from build123d import *

# Parameters (mm, degrees)
SKETCH1_W           = 75
SKETCH1_H           = 45
SKETCH1_R           = 14
SKETCH1_R_2         = 1.6
BOSS_EXTRUDE1_DEPTH = 2.032
FILLET2_R           = 5
SKETCH2_R           = 1.6
CUT_EXTRUDE1_DEPTH  = 3.032
SKETCH3_R           = 1.6
CUT_EXTRUDE2_DEPTH  = 3.032


with BuildPart() as part:
    # Sketch1 → Boss-Extrude1 (new body)
    with BuildSketch(Plane.XY):
        Rectangle(SKETCH1_W, SKETCH1_H)
        Circle(SKETCH1_R, mode=Mode.SUBTRACT)
        with Locations((-15.5, 15.5)):
            Circle(SKETCH1_R_2, mode=Mode.SUBTRACT)
        with Locations((15.5, 15.5)):
            Circle(SKETCH1_R_2, mode=Mode.SUBTRACT)
        with Locations((15.5, -15.5)):
            Circle(SKETCH1_R_2, mode=Mode.SUBTRACT)
        with Locations((-15.5, -15.5)):
            Circle(SKETCH1_R_2, mode=Mode.SUBTRACT)
    extrude(amount=BOSS_EXTRUDE1_DEPTH)

    # Fillet2
    fillet2_edges = [part.edges().sort_by_distance(p)[0] for p in [
        (37.5, -22.5, 1.016),
        (-37.5, -22.5, 1.016),
        (-37.5, 22.5, 1.016),
        (37.5, 22.5, 1.016),
    ]]
    fillet(fillet2_edges, radius=FILLET2_R)

    # Sketch2 → Cut-Extrude1 (cut, through all)
    with BuildSketch(Plane.XY.offset(2.032)):
        with Locations((-30, 0)):
            Circle(SKETCH2_R)
        with Locations((-30, 15)):
            Circle(SKETCH2_R)
        with Locations((-30, -15)):
            Circle(SKETCH2_R)
        with Locations((30, -15)):
            Circle(SKETCH2_R)
        with Locations((30, 15)):
            Circle(SKETCH2_R)
        with Locations((30, 0)):
            Circle(SKETCH2_R)
    extrude(amount=-CUT_EXTRUDE1_DEPTH, mode=Mode.SUBTRACT)

    # Sketch3 → Cut-Extrude2 (cut, through all)
    with BuildSketch(Plane(origin=(0, 0, 0), x_dir=(-1, 0, 0), z_dir=(0, 0, -1))):
        with Locations((-32.5, 5)):
            Circle(SKETCH3_R)
        with Locations((-32.5, -5)):
            Circle(SKETCH3_R)
        with Locations((32.5, -5)):
            Circle(SKETCH3_R)
        with Locations((32.5, 5)):
            Circle(SKETCH3_R)
    extrude(amount=-CUT_EXTRUDE2_DEPTH, mode=Mode.SUBTRACT)


solid = part.part
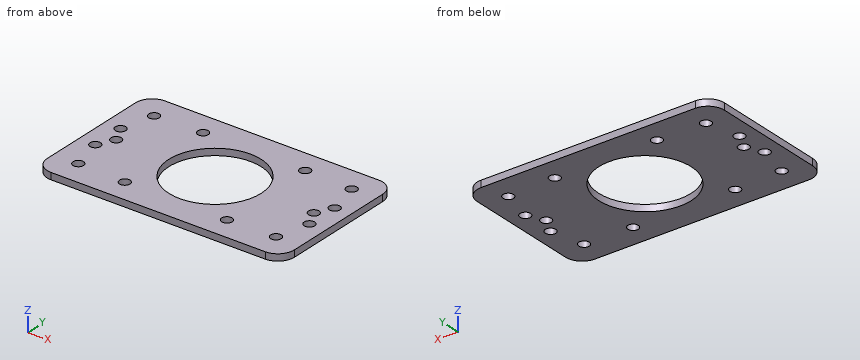
Geometry check sheet. Reference: the model listing, model coordinates, mm. Give positions to 0.01 mm unless a question says otherwise; leave off trailing zeros. Write each loop counter-clockwise with the first axis right and the second up, starting at its lowest first coordinate (ties: lowest second). Pieces come first, ordered by that corner, then holes. Notation, with made-up numbers: (-37.5, 23.25) - (-9.5, 23.25) arc R11 ccw to (-9.5, 34.25) - close; hole circle Ø8 at (72, 30.5). An arc over 180 degrees is marked (long way). Put each result on its own line as item: value.
1. Go/stop test with a flat-tipped pin: pin 1 (3 mm diameter, centred on x = 30, y = 0, fed in from +Z). Record where the tip stops, or that it passes through.
Ans:
pin 1: passes through
2. Sectioned sample at B-B, the plane x = 15.5. Enter the section's corners in (y, z).
Ans:
outline: (-22.5, 0) - (-17.1, 0) - (-17.1, 2.03) - (-22.5, 2.03) - close; (-13.9, 0) - (13.9, 0) - (13.9, 2.03) - (-13.9, 2.03) - close; (17.1, 0) - (22.5, 0) - (22.5, 2.03) - (17.1, 2.03) - close
3. Sectioned sample at A-A, the plane y = 0. Enter the section's corners in (x, z), plus the area to 3 significant figures.
Ans:
outline: (-37.5, 0) - (-31.6, 0) - (-31.6, 2.03) - (-37.5, 2.03) - close; (-28.4, 0) - (-14, 0) - (-14, 2.03) - (-28.4, 2.03) - close; (14, 0) - (28.4, 0) - (28.4, 2.03) - (14, 2.03) - close; (31.6, 0) - (37.5, 0) - (37.5, 2.03) - (31.6, 2.03) - close
area: 82.5 mm²
4. Thickness scan on line 1 (Y direction, x = -15.5, z = 0.7); line 2 (Y direction, x = -32.5, z = 1.1); line 3 (Y direction, x = 0, z = 0.6). Record the ranges inside material, lowest first.
Ans:
line 1: y = -22.5 to -17.1, -13.9 to 13.9, 17.1 to 22.5
line 2: y = -22.5 to -6.6, -3.4 to 3.4, 6.6 to 22.5
line 3: y = -22.5 to -14, 14 to 22.5
5. Sectioned sample at C-C, the plane x = 0. Enter the section's corners in (y, z).
Ans:
outline: (-22.5, 0) - (-14, 0) - (-14, 2.03) - (-22.5, 2.03) - close; (14, 0) - (22.5, 0) - (22.5, 2.03) - (14, 2.03) - close
6. Sectioned sample at D-D, the plane x = 30. Enter the section's corners in (y, z).
Ans:
outline: (-22.5, 0) - (-16.6, 0) - (-16.6, 2.03) - (-22.5, 2.03) - close; (-13.4, 0) - (-1.6, 0) - (-1.6, 2.03) - (-13.4, 2.03) - close; (1.6, 0) - (13.4, 0) - (13.4, 2.03) - (1.6, 2.03) - close; (16.6, 0) - (22.5, 0) - (22.5, 2.03) - (16.6, 2.03) - close
